Verification items for the finished model (mm, model axes). Face numbers are marked on the shaded views. Give positions to 0.01 mm unless a question says otherwise; leave off trailing zeros. Loops run counter-clockwise (first coordinate to the right, second up) from the corner with the lowest first, then second, coordinate; pieces in that order, holes last. Notation, with made-up numbers: (-30.75, -20) - (-5.75, -20) arc R9 ccw to (-5.75, -9) - close; hole circle Ø10 at (-12, 23). An arc over 180 degrees is marked (long way). Answer in a Markdown table with one row per item.
```python
from build123d import *

# Parameters (mm, degrees)
SKETCH1_W           = 100
SKETCH1_H           = 50
SKETCH1_W_2         = 3
SKETCH1_H_2         = 20
BOSS_EXTRUDE1_DEPTH = 3
SKETCH1_3_W         = 3
SKETCH1_3_H         = 20
BOSS_EXTRUDE2_DEPTH = 37
SKETCH1_4_W         = 3
SKETCH1_4_H         = 20
BOSS_EXTRUDE3_DEPTH = 31.4
SKETCH2_R           = 3
SKETCH2_R_2         = 1.1
CUT_EXTRUDE1_DEPTH  = 3
CIRPATTERN1_COUNT   = 4
SKETCH3_R           = 1.6
CUT_EXTRUDE2_DEPTH  = 15


with BuildPart() as part:
    # Sketch1 → Boss-Extrude1 (new body)
    with BuildSketch(Plane(origin=(0, 0, 0), x_dir=(1, 0, 0), z_dir=(0, 1, 0))):
        Rectangle(SKETCH1_W, SKETCH1_H)
        with Locations((-36.5, 0)):
            Rectangle(SKETCH1_W_2, SKETCH1_H_2, mode=Mode.SUBTRACT)
        with Locations((6.05, 0)):
            Rectangle(SKETCH1_W_2, SKETCH1_H_2, mode=Mode.SUBTRACT)
    extrude(amount=BOSS_EXTRUDE1_DEPTH)

    # Sketch1<3> → Boss-Extrude2 (add)
    with BuildSketch(Plane(origin=(0, 0, 0), x_dir=(1, 0, 0), z_dir=(0, 1, 0))):
        with Locations((6.05, 0)):
            Rectangle(SKETCH1_3_W, SKETCH1_3_H)
    extrude(amount=BOSS_EXTRUDE2_DEPTH)

    # Sketch1<4> → Boss-Extrude3 (add)
    with BuildSketch(Plane(origin=(0, 0, 0), x_dir=(1, 0, 0), z_dir=(0, 1, 0))):
        with Locations((-36.5, 0)):
            Rectangle(SKETCH1_4_W, SKETCH1_4_H)
    extrude(amount=BOSS_EXTRUDE3_DEPTH)

    # Sketch2 → Cut-Extrude1 (cut)
    with BuildSketch(Plane(origin=(7.55, 0, 0), x_dir=(0, 0, -1), z_dir=(1, 0, 0))):
        with Locations((0, 27)):
            Circle(SKETCH2_R)
        with Locations((5.656854249, 32.656854249)):
            Circle(SKETCH2_R_2)
    cut_extrude1 = extrude(amount=-CUT_EXTRUDE1_DEPTH, mode=Mode.SUBTRACT)

    # CirPattern1: Cut-Extrude1 ×4 about axis
    cirpattern1_axis = Axis((0, 27, 0), (1, 0, 0))
    for i in range(1, CIRPATTERN1_COUNT):
        add(cut_extrude1.rotate(cirpattern1_axis, i * 360 / CIRPATTERN1_COUNT), mode=Mode.SUBTRACT)

    # Sketch3 → Cut-Extrude2 (cut)
    with BuildSketch(Plane.ZY.offset(50)):
        with Locations((0, 27)):
            Circle(SKETCH3_R)
    extrude(amount=-CUT_EXTRUDE2_DEPTH, mode=Mode.SUBTRACT)


solid = part.part
```
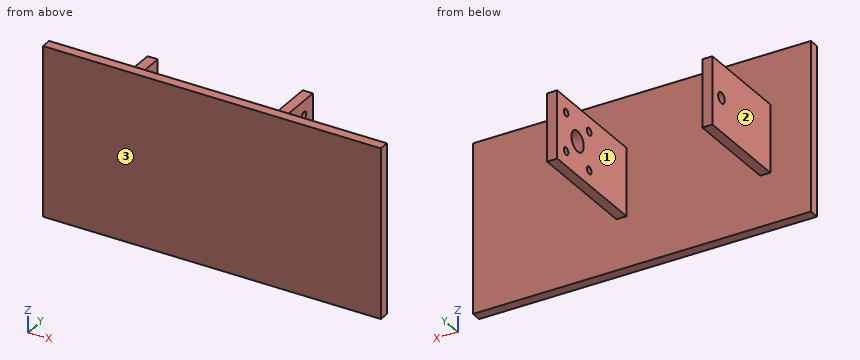
Q1. Sectioned sample at B-B (z = 0). Record the cut outline in (x, y).
Completed:
| item | result |
|---|---|
| outline | (-50, 0) - (50, 0) - (50, 3) - (7.55, 3) - (7.55, 24) - (4.55, 24) - (4.55, 3) - (-35, 3) - (-35, 25.4) - (-38, 25.4) - (-38, 3) - (-50, 3) - close; (-38, 28.6) - (-35, 28.6) - (-35, 31.4) - (-38, 31.4) - close; (4.55, 30) - (7.55, 30) - (7.55, 37) - (4.55, 37) - close |
Q2. Draft check along X on the marked faces 1, 2 and 3. Enter one of: +X half, -X half, draft (parallel to the pull), parting line (faces both ways), or undercut.
Completed:
| item | result |
|---|---|
| face 1 | undercut |
| face 2 | -X half |
| face 3 | draft |
Q3. Sectioned sample at A-A (y = 27). Record the cut outline in (x, z), and give its area (3 significant figures).
Completed:
| item | result |
|---|---|
| outline | (-38, -10) - (-35, -10) - (-35, -1.6) - (-38, -1.6) - close; (-38, 1.6) - (-35, 1.6) - (-35, 10) - (-38, 10) - close; (4.55, -10) - (7.55, -10) - (7.55, -3) - (4.55, -3) - close; (4.55, 3) - (7.55, 3) - (7.55, 10) - (4.55, 10) - close |
| area | 92.4 mm^2 |
Q4. Sectioned sample at C-C (y = 8.5). Record the cut outline in (x, z), and give its area (3 significant figures).
Completed:
| item | result |
|---|---|
| outline | (-38, -10) - (-35, -10) - (-35, 10) - (-38, 10) - close; (4.55, -10) - (7.55, -10) - (7.55, 10) - (4.55, 10) - close |
| area | 120 mm^2 |
Q5. Sectioned sample at D-D (x = -13). Record the cut outline in (y, z).
Completed:
| item | result |
|---|---|
| outline | (0, -25) - (3, -25) - (3, 25) - (0, 25) - close |
Q6. Thickness scan on line 1 (X direction, y = 14, z = -0.5); line 2 (Y direction, x = 38, z = -9.5); line 3 (Z direction, x = 6.2, y = 27). Record the ranges inside material, lowest first.
Completed:
| item | result |
|---|---|
| line 1 | -38 to -35, 4.55 to 7.55 |
| line 2 | 0 to 3 |
| line 3 | -10 to -3, 3 to 10 |
Q7. Go/stop test with flat-tipped pins: P1, Ø10, axis at y = 21.5, z = 4.5, coming from the -X side; P2, Ø5, axis at y = 27, z = 0, coming from the +X side; P3, Ø8, axis at x = -10.5, z = -14.5, coming from the +Y side. Record where each tip stops, or that it passes through.
Completed:
| item | result |
|---|---|
| P1 | x = -38 |
| P2 | x = -35 |
| P3 | y = 3 |
